from build123d import *

# Parameters (mm, degrees)
F2_SIZE2 = 9.99999
F2_SIZE  = 9.99999
F3_SIZE2 = 3
F3_SIZE  = 3


# Not quite as in the source:
# - a fillet or chamfer is up to 0.001 mm smaller than in the source, because OpenCascade refuses the exact size


with BuildPart() as f1:
    # F0 (on Right) → F1 (revolve)
    with BuildSketch(Plane.YZ):
        Polygon((0, 0), (160, 0), (160, 40), (150, 40), (150, 20), (25, 20), (25, 7.5), (0, 7.5), align=None)
    revolve(axis=Axis((0, 80, 0), (0, 1, 0)))

    # F2 (size 10 and 10 in the source; OpenCascade refuses exactly that, so slightly less here)
    f2_edges = [f1.edges().sort_by_distance(p)[0] for p in [
        (0, 160, -40),
    ]]
    chamfer(f2_edges, length=F2_SIZE, length2=F2_SIZE2)

    # F3
    f3_edges = [f1.edges().sort_by_distance(p)[0] for p in [
        (0, 25, -20),
    ]]
    chamfer(f3_edges, length=F3_SIZE, length2=F3_SIZE2)


solid = f1.part
Can you work these out from the model? Positions are in its coordinate system, mm. A direction names the side the tool comes from. Round coordinates to 2 decimals unless told otherwise and drop trailing zeros. Order: outer loops, then holes, each group sorted by start corner. A loop starts at its lowest first (then second) coordinate and runs counter-clockwise, first axis right, second up. Notation, with made-up numbers: M -1,53 L 52,53 A22 ccw 52,71 Z; hole C 9,0.25 d9. An arc over 180 degrees is marked long. Use a Markdown table: item, result.
1) If I drill on line 1 along Z through (x, y) = (-0.5, 101); line 2 along Y through (x, z) = (21, -7); line 3 along Y through (x, z) = (12, 0), over which ranges is the centre line in solid material (lowest first)?
Geometry says:
| item | result |
|---|---|
| line 1 | z = -19.99 to 19.99 |
| line 2 | y = 150 to 160 |
| line 3 | y = 25 to 160 |
2) Imagine slicing it at C-C (y = 135). List the corners of the cut face in (x, z) for me.
Geometry says:
| item | result |
|---|---|
| outline | C 0,0 d40 |
3) On a 3-axis mill with a long thin cutter (end or side, diameter ignored), from which of +Z, -Z, +X, -X, +Y, -Y can I reach the whole of each face in a straight line? I mean faces 1 (the face through (-19.524, 88.146, -4.336)), 2 (the face through (30.365, 159.374, -3.987)). Say none if no direction works.
Geometry says:
| item | result |
|---|---|
| face 1 | -Y |
| face 2 | +Y |
4) I'm going to push flat-ended pins straight in: P1, Ø6, axis at x = 30, z = 4, coming from the -Y side; P2, Ø8, axis at x = -7, y = 46, coming from the +Z side; P3, Ø6, axis at x = -16.5, z = -29, coming from the +Y side. Where does each tip first touch, or does it pass through?
Geometry says:
| item | result |
|---|---|
| P1 | stops at y = 150 |
| P2 | stops at z = 19.77 |
| P3 | stops at y = 159.63 |
